Job drawing, mm, ordinate dimensions from the low corner. One solid piece. A direction names the side the tool comes from. Round coordinates to 2 decimals unless told otherwise and drop trailing zeros. Loops run counter-clockwise (first coordinate to the right, second up) from the corner with the lowest first, then second, coordinate; pieces in that order, holes last.
1) Band-saw the part on A-A, the plane x = 10.5. Write the cut outline in (y, z), then the cut area to 3 significant figures.
2) Drop a flat-ended pin along its axis: P1, Ø3, axis at x = 10.5, z = 30, coming from the +Y side. Give the stop position or say it passes through.
3) Band-saw the part on B-B, the plane z = 30. Write the cut outline in (x, y).
4) 3-axis set-ups, long thin cutter, end or side, ignore diameter. For the marked faces 1 and 2: which of +Z, -Z, +X, -X, +Y, -Y reach the whole face in a straight line?
5) Mould opens along X. For the marked faces 3, 4, 5 and 6 say: +X half, -X half, draft (parallel to the pull), parting line (faces both ways), or undercut.
6) Band-saw the part on C-C, the plane y = 15. Write the cut outline in (x, z).
7) Band-saw the part on D-D, the plane z = 21.5. Write the cut outline in (x, y), then the cut area to 3 significant figures.
8) Probe line 1 (X direction, y = 1.4, z = 30); line 2 (X direction, y = 11.5, z = 57); line 3 (Z direction, x = 43, y = 5.5). List the from-to ranges inside material, lowest first.
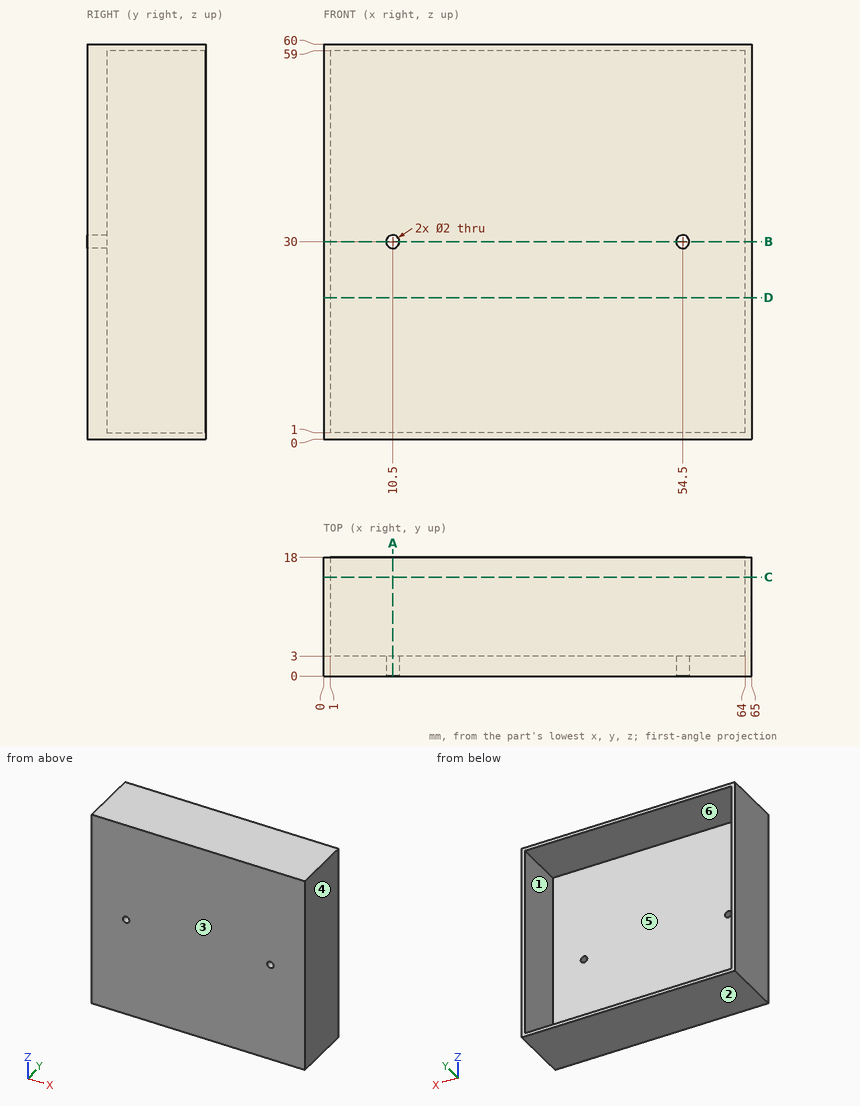
Reported:
1. outline: (0, 0) - (18, 0) - (18, 1) - (3, 1) - (3, 29) - (0, 29) - close; (0, 31) - (3, 31) - (3, 59) - (18, 59) - (18, 60) - (0, 60) - close
1. area: 204 mm2
2. P1: stops at y = 3
3. outline: (0, 0) - (9.5, 0) - (9.5, 3) - (1, 3) - (1, 18) - (0, 18) - close; (11.5, 0) - (53.5, 0) - (53.5, 3) - (11.5, 3) - close; (55.5, 0) - (65, 0) - (65, 18) - (64, 18) - (64, 3) - (55.5, 3) - close
4. face 1: +Y
4. face 2: -Z, +X, -X, +Y, -Y
5. face 3: draft
5. face 4: +X half
5. face 5: undercut
5. face 6: undercut
6. outline: (0, 0) - (65, 0) - (65, 60) - (0, 60) - close; hole (1, 1) - (64, 1) - (64, 59) - (1, 59) - close
7. outline: (0, 0) - (65, 0) - (65, 18) - (64, 18) - (64, 3) - (1, 3) - (1, 18) - (0, 18) - close
7. area: 225 mm2
8. line 1: x = 0 to 9.5, 11.5 to 53.5, 55.5 to 65
8. line 2: x = 0 to 1, 64 to 65
8. line 3: z = 0 to 1, 59 to 60
